Here's how the part is built. I have some questions about the finished solid (model axes, mm). A direction names the side the tool comes from. Round coordinates to 2 decimals unless told otherwise and drop trailing zeros. Loops run counter-clockwise (first coordinate to the right, second up) from the corner with the lowest first, then second, coordinate; pieces in that order, holes last. Notation, with made-up numbers: M -33,-20.5 L 25,-20.5 A33 ccw 25,14.5 Z; hole C -31,39.25 d2. An arc over 180 degrees is marked long. Write item = value, one per line. Start each with the question number.
from build123d import *

# Parameters (mm, degrees)
SKETCH1_W              = 61.48
SKETCH1_H              = 61.48
SKETCH1_R              = 2.55
SKETCH1_R_2            = 19.812
BOSS_EXTRUDE1_DEPTH    = 5.08
FILLET1_R              = 2.54
BOSS_EXTRUDE2_DEPTH    = 5.08
FILLET2_R              = 2.54
F_10_CLEARANCE_HOLE1_D = 5.1054


with BuildPart() as part:
    # Sketch1 → Boss-Extrude1 (new body)
    with BuildSketch(Plane.XY):
        Rectangle(SKETCH1_W, SKETCH1_H)
        with Locations((-23.570000148, 23.570000149)):
            Circle(SKETCH1_R, mode=Mode.SUBTRACT)
        with Locations((23.569999852, 23.570000149)):
            Circle(SKETCH1_R, mode=Mode.SUBTRACT)
        with Locations((23.569999852, -23.569999851)):
            Circle(SKETCH1_R, mode=Mode.SUBTRACT)
        with Locations((-23.570000148, -23.569999851)):
            Circle(SKETCH1_R, mode=Mode.SUBTRACT)
        with Locations((-1.48e-07, 1.49e-07)):
            Circle(SKETCH1_R_2, mode=Mode.SUBTRACT)
    extrude(amount=-BOSS_EXTRUDE1_DEPTH)

    # Fillet1
    fillet1_edges = [part.edges().sort_by_distance(p)[0] for p in [
        (-30.74, 30.74, -2.54),
        (30.74, 30.74, -2.54),
        (30.74, -30.74, -2.54),
        (-30.74, -30.74, -2.54),
    ]]
    fillet(fillet1_edges, radius=FILLET1_R)

    # Sketch7 → Boss-Extrude2 (add, through all)
    with BuildSketch(Plane.XY):
        with BuildLine():
            Line((-27.259871939, -36.240128061), (-21.759743879, -30.74))
            Line((-21.759743879, -30.74), (-30.74, -21.759743879))
            Line((-30.74, -21.759743879), (-36.240128061, -27.259871939))
            ThreePointArc((-36.240128061, -27.259871939), (-36.240128061, -36.240128061), (-27.259871939, -36.240128061))
        make_face()
        with BuildLine():
            Line((30.74, -21.759743879), (21.759743879, -30.74))
            Line((21.759743879, -30.74), (27.259871939, -36.240128061))
            ThreePointArc((27.259871939, -36.240128061), (36.240128061, -36.240128061), (36.240128061, -27.259871939))
            Line((36.240128061, -27.259871939), (30.74, -21.759743879))
        make_face()
    extrude(amount=-BOSS_EXTRUDE2_DEPTH)

    # Fillet2
    fillet2_edges = [part.edges().sort_by_distance(p)[0] for p in [
        (-30.74, -21.759743879, -2.54),
        (-21.759743879, -30.74, -2.54),
        (21.759743879, -30.74, -2.54),
        (30.74, -21.759743879, -2.54),
    ]]
    fillet(fillet2_edges, radius=FILLET2_R)

    # #10 Clearance Hole1 (through all)
    with Locations(Plane.XY):
        with Locations((-31.75, -31.75), (31.75, -31.75)):
            Hole(F_10_CLEARANCE_HOLE1_D / 2)


solid = part.part
Item 1: I want a section at A-A, the plane x = 0. List the corners of the cut face in (y, z) for me.
Item 2: Please list where these lines run through material, in increasing order: line 1 (X direction, y = -31.5, z = -0.55); line 2 (Y direction, x = -23.57, z = -2.4); line 3 (X direction, y = -29.5, z = -1.5). Write a range as [from, to].
Item 3: Will these pins go through, and if not, where does the flat tip stop? pin 1 Ø4.5 at (x, y) = (23.57, -23.57) entering from +Z; pin 2 Ø1.5 at (y, z) = (-1, -3.5) entering from -X; pin 3 Ø2 at (y, z) = (14.5, -3.5) entering from +X; pin 4 Ø2 at (x, z) = (-25.5, -3) entering from -Y.
Item 4: For faces 5 (the cylindrical face through (-21.693, -30.939, -2.576)), 6 (the cylindrical face through (36.14, -36.34, -2.5)), which set-ups out of +Z, -Z, +X, -X, +Y, -Y let a thin tool reach every point of the face, with its end or its side?
Item 5: I want a section at D-D, the plane y = -23.57. List the corners of the cut face in (x, z) for me, then the cut area to 3 significant figures.
Item 6: I want a section at C-C, the plane x = 23.57. List the corners of the cut face in (y, z) for me, then the cut area to 3 significant figures.
Item 7: We'd pull the mould along X, two halves only. Please class faces 1 (the cylindrical face through (-30.939, -21.693, -2.576)), 2 (the cylindrical face through (29.392, -32.728, -2.576)), 3 (the flat face through (30.74, 3, -3)), 4 (the cylindrical face through (21.69, 25.29, -2.5)): released by +X, released by -X, zero draft, split by the parting line, or undercut.
Worked out:
q1.outline = M -30.74,-5.08 L -19.81,-5.08 L -19.81,0 L -30.74,0 Z; M 19.81,-5.08 L 30.74,-5.08 L 30.74,0 L 19.81,0 Z
q2.line_1 = [-38.1, -34.29], [-29.21, -22.52], [22.52, 29.21], [34.29, 38.1]
q2.line_2 = [-32.55, -26.12], [-21.02, 21.02], [26.12, 30.74]
q2.line_3 = [-37.69, -32.96], [-30.54, 30.54], [32.96, 37.69]
q3.pin_1 = through
q3.pin_2 = -30.74
q3.pin_3 = 30.74
q3.pin_4 = -35.48
q4.face_5 = +Z, -Z, -Y
q4.face_6 = +Z, -Z
q5.outline = M -32.55,-5.08 L -26.12,-5.08 L -26.12,0 L -32.55,0 Z; M -21.02,-5.08 L 21.02,-5.08 L 21.02,0 L -21.02,0 Z; M 26.12,-5.08 L 32.55,-5.08 L 32.55,0 L 26.12,0 Z
q5.area = 279 mm2
q6.outline = M -32.55,-5.08 L -26.12,-5.08 L -26.12,0 L -32.55,0 Z; M -21.02,-5.08 L 21.02,-5.08 L 21.02,0 L -21.02,0 Z; M 26.12,-5.08 L 30.74,-5.08 L 30.74,0 L 26.12,0 Z
q6.area = 270 mm2
q7.face_1 = released by -X
q7.face_2 = undercut
q7.face_3 = released by +X
q7.face_4 = undercut
